Read the model definition and answer for the solid it produces. Units are mm, in the model's axes. Coordinates: 2 decimals unless noted, no trailing zeros. Write each loop counter-clockwise with the first axis right and the second up, starting at its lowest first coordinate (ties: lowest second). Pieces come first, ordered by that corner, then holes.
(1) Section D-D on z = 30 is taken. Write down the section's boundary in (x, y), then the cut area to 3 significant figures.
(2) Section A-A on x = 3.25 is taken. Write down the section's boundary in (y, z), then the cut area to 4 significant figures.
(3) Find the intervals of material crossed by probe 1 along Z at (x, y) = (2, 1.05); probe 2 along X at (y, z) = (2.3, 5); probe 3 along Z at (x, y) = (14.5, 1.2), in increasing order.
(4) Section C-C on x = 20.5 is taken. Write down the section's boundary in (y, z).
(5) Section B-B on y = 0.85 is taken. Write down the section's boundary in (x, z).
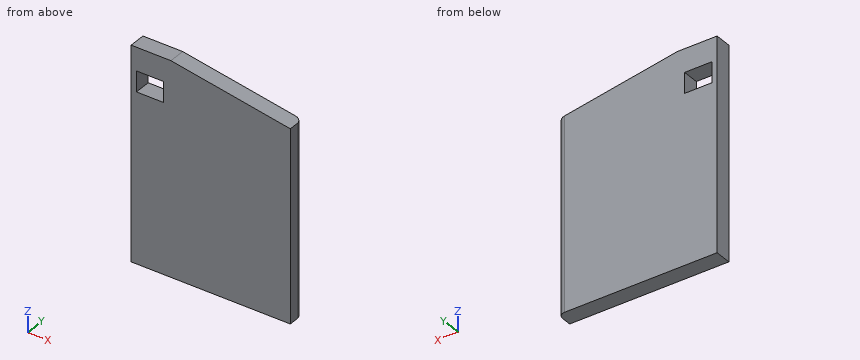
from build123d import *

# Parameters (mm, degrees)
SKETCH_3_W          = 2.5
SKETCH_3_H          = 24
EXTRUDE_1_DEPTH     = 33
FILLET_1_R          = 1
CUT_EXTRUDE_1_DEPTH = 41.880924647
SKETCH_5_W          = 2.5
SKETCH_5_H          = 3.1
CUT_EXTRUDE_2_DEPTH = 4.9
SKETCH_6_W          = 24
SKETCH_6_H          = 2.5
CUT_EXTRUDE_3_DEPTH = 1
CUT_EXTRUDE_4_DEPTH = 41.078048855
SKETCH_8_W          = 0.8
SKETCH_8_H          = 3.1
EXTRUDE_2_DEPTH     = 2.5


with BuildPart() as part:
    # 草图3 → 凸台-拉伸1 (new body)
    with BuildSketch(Plane(origin=(0, 0, 0), x_dir=(0, 1, 0), z_dir=(0, 0, 1))):
        with Locations((1.25, -12)):
            Rectangle(SKETCH_3_W, SKETCH_3_H)
    extrude(amount=EXTRUDE_1_DEPTH)

    # 圆角1
    fillet_1_edges = [part.edges().sort_by_distance(p)[0] for p in [
        (24, 2.5, 16.5),
    ]]
    fillet(fillet_1_edges, radius=FILLET_1_R)

    # 草图4 → 切除-拉伸1 (cut, through all)
    with BuildSketch(Plane.XZ):
        Polygon((3, 33), (24, 31.162738066), (24, 33), align=None)
    extrude(amount=-CUT_EXTRUDE_1_DEPTH, mode=Mode.SUBTRACT)

    # 草图5 → 切除-拉伸2 (cut)
    with BuildSketch(Plane(origin=(0, 0, 0), x_dir=(0, -1, 0), z_dir=(-1, 0, 0))):
        with Locations((-1.25, 26.95)):
            Rectangle(SKETCH_5_W, SKETCH_5_H)
    extrude(amount=-CUT_EXTRUDE_2_DEPTH, mode=Mode.SUBTRACT)

    # 草图6 → 切除-拉伸3 (cut)
    with BuildSketch(Plane.XY.offset(33)):
        with Locations((12, 1.25)):
            Rectangle(SKETCH_6_W, SKETCH_6_H)
    extrude(amount=-CUT_EXTRUDE_3_DEPTH, mode=Mode.SUBTRACT)

    # 草图7 → 切除-拉伸4 (cut, through all)
    with BuildSketch(Plane.XZ):
        Polygon((24, 31.162738066), (24, 28.826114347), (6, 32), (14.430052303, 32), align=None)
    extrude(amount=-CUT_EXTRUDE_4_DEPTH, mode=Mode.SUBTRACT)

    # 草图8 → 凸台-拉伸2 (add)
    with BuildSketch(Plane(origin=(0, 2.5, 0), x_dir=(-1, 0, 0), z_dir=(0, 1, 0))):
        with Locations((-0.4, 26.95)):
            Rectangle(SKETCH_8_W, SKETCH_8_H)
    extrude(amount=-EXTRUDE_2_DEPTH)


solid = part.part
Response:
1. outline: (0, 0) - (17.34, 0) - (17.34, 2.5) - (0, 2.5) - close
1. area: 43.4 mm2
2. outline: (0, 0) - (2.5, 0) - (2.5, 25.4) - (0, 25.4) - close; (0, 28.5) - (2.5, 28.5) - (2.5, 32) - (0, 32) - close
2. area: 72.25 mm2
3. probe 1: z = 0 to 25.4, 28.5 to 32
3. probe 2: x = 0 to 23.6
3. probe 3: z = 0 to 30.5
4. outline: (0, 0) - (2.5, 0) - (2.5, 29.44) - (0, 29.44) - close
5. outline: (0, 0) - (24, 0) - (24, 28.83) - (6, 32) - (0, 32) - close; hole (0.8, 25.4) - (4.9, 25.4) - (4.9, 28.5) - (0.8, 28.5) - close
